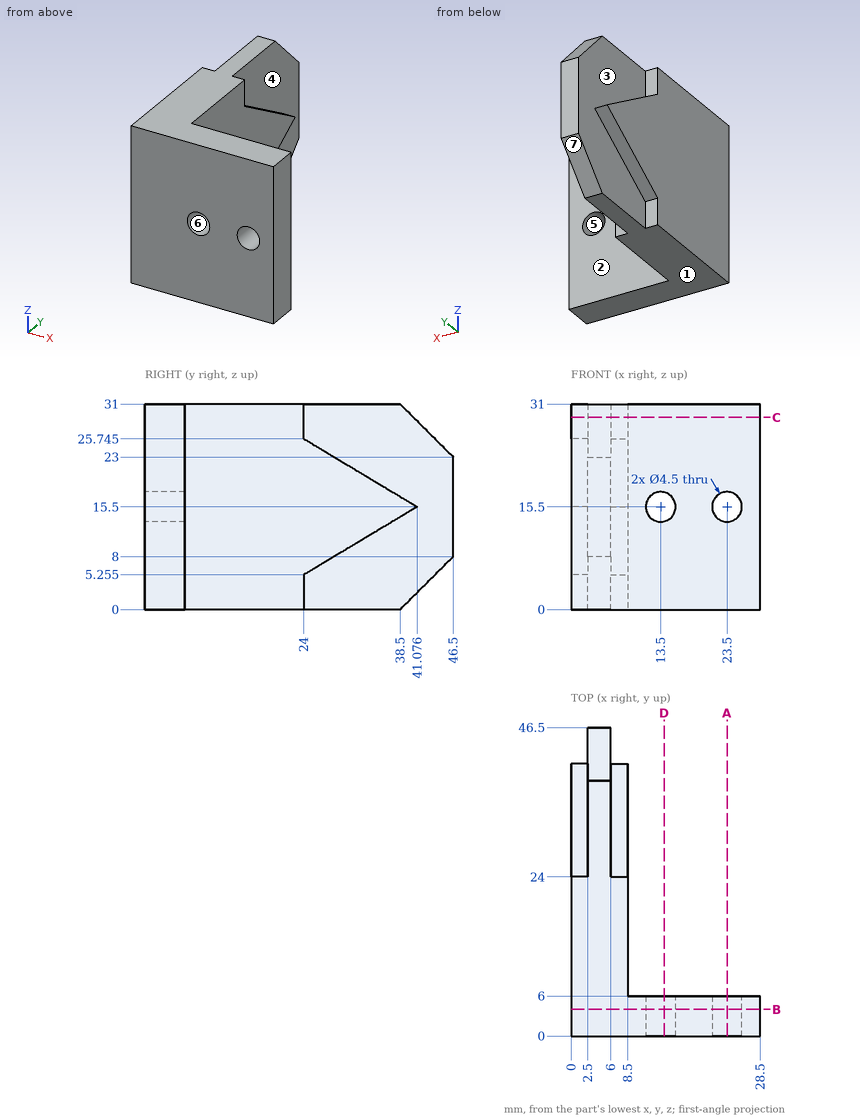
Answer from the drawing. Dimensions are ordinates in mm from the lowest x, y and z of the part. A direction names the side the tool comes from. Round coordinates to 2 decimals unless told otherwise and drop trailing zeros. Write each loop counter-clockwise with the first axis right and the second up, starting at its lowest first coordinate (ties: lowest second). Pieces come first, ordered by that corner, then holes. Notation, with made-up numbers: (55, 9) - (82, 9) arc R23 cw to (82, 23) - close; hole circle Ø1 at (19, -28.5). An arc over 180 degrees is marked (long way). One line per item, written item: value.
Q1. Find section D-D (x = 14). Determine the outline of the cut face in (y, z), and give its area (3 significant figures).
The answers:
outline: (0, 0) - (6, 0) - (6, 13.31) - (0, 13.31) - close; (0, 17.69) - (6, 17.69) - (6, 31) - (0, 31) - close
area: 160 mm2
Q2. Which of the six approach directions +Z, -Z, +X, -X, +Y, -Y give full straight-line access (tool end or side, diameter ignored) to the marked faces 1, 2 and 3?
The answers:
face 1: -Z, +X, -X, +Y, -Y
face 2: +Z, -Z, +X, +Y
face 3: -X, +Y
Q3. Find section C-C (z = 29). Determine the outline of the cut face in (x, y), and give its area (3 significant figures).
The answers:
outline: (0, 0) - (28.5, 0) - (28.5, 6) - (8.5, 6) - (8.5, 24) - (6, 24) - (6, 40.5) - (2.5, 40.5) - (2.5, 24) - (0, 24) - close
area: 382 mm2
Q4. Find section A-A (x = 23.5). Determine the outline of the cut face in (y, z).
The answers:
outline: (0, 0) - (6, 0) - (6, 13.25) - (0, 13.25) - close; (0, 17.75) - (6, 17.75) - (6, 31) - (0, 31) - close
Q5. Straight lines are drawn through the part: line 1 (Z direction, x = 23.5, y = 3.3); line 2 (X direction, y = 3, z = 15) (1 decimal); line 3 (Y direction, x = 18.75, z = 23). For each, find the intervals that lie inside material, in ascending order. Write a range as from..to.
The answers:
line 1: z = 0..13.25, 17.75..31
line 2: x = 0..11.3, 15.7..21.3, 25.7..28.5
line 3: y = 0..6
Q6. Each of these flat-tipped pins is pushed along its axis until it touches: P1, Ø4, axis at x = 23.5, z = 15.5, coming from the +Y side; P2, Ø15.5, axis at y = 32.5, z = 17, coming from the +X side; P3, Ø6, axis at x = 13.5, z = 15.5, coming from the +Y side; P4, Ø3, axis at x = 1.5, z = 2, coming from the +Y side. Where does it stop, or does it pass through?
The answers:
P1: passes through
P2: stops at x = 8.5
P3: stops at y = 6
P4: stops at y = 41.62
Q7. Find section B-B (y = 4). Determine the outline of the cut face in (x, z), and give its area (3 significant figures).
The answers:
outline: (0, 0) - (28.5, 0) - (28.5, 31) - (0, 31) - close; hole circle Ø4.5 at (13.5, 15.5); hole circle Ø4.5 at (23.5, 15.5)
area: 852 mm2
Q8. For a pull along Z with two mould halves and no side action, classify the marked faces 4, 5, 6 and 7 as pulls with the +Z half, pulls with the -Z half, needs draft (parallel to the pull), parting line crosses it, or undercut.
The answers:
face 4: needs draft
face 5: undercut
face 6: undercut
face 7: pulls with the -Z half
